from build123d import *

# Parameters (mm, degrees)
PAD014_DEPTH         = 3
SKETCH055_R          = 1.7
POCKET019_DEPTH      = 364.282338
POCKET019_DEPTH_BACK = 367.282338


with BuildPart() as part:
    # Sketch052 → Pad014 (new body)
    with BuildSketch(Plane.XY):
        with BuildLine():
            ThreePointArc((152.959511, 127.101705), (84.480895, 180.040089), (0, 198.875477))
            Line((0, 198.875477), (0, 208.875477))
            ThreePointArc((160.650731, 133.492724), (88.728824, 189.092995), (0, 208.875477))
            ThreePointArc((152.959511, 127.101705), (160.000631, 126.451604), (160.650731, 133.492724))
        make_face()
    pad014 = extrude(amount=PAD014_DEPTH)

    # Sketch055 → Pocket019 (cut, two sides)
    with BuildSketch(Plane.XY) as pocket019_sk:
        with Locations((143.11, 145.205847)):
            Circle(SKETCH055_R)
        with BuildLine():
            Line((0, 202.175477), (0, 205.575477))
            ThreePointArc((0, 202.175477), (1.7, 203.875477), (0, 205.575477))
        make_face()
    pocket019 = extrude(amount=-POCKET019_DEPTH, mode=Mode.SUBTRACT) + extrude(pocket019_sk.sketch, amount=POCKET019_DEPTH_BACK, mode=Mode.SUBTRACT)

    # Mirrored019: Pad014, Pocket019 across Sketch052 V_Axis
    add(pad014.mirror(Plane(origin=(0, 0, 0), x_dir=(0, 0, 1), z_dir=(1, 0, 0))))
    add(pocket019.mirror(Plane(origin=(0, 0, 0), x_dir=(0, 0, 1), z_dir=(1, 0, 0))), mode=Mode.SUBTRACT)


solid = part.part
Geometry: final body of the model. Coordinates: model frame, mm. Round coordinates to 2 decimals unless told otherwise and drop trailing zeros. Loops run counter-clockwise (first coordinate to the right, second up) from the corner with the lowest first, then second, coordinate; pieces in that order, holes last. Notation, with made-up numbers: (17.25, -30.5) -> (26.25, -30.5) arc R26 cw to (26.25, -2.5) -> close; hole circle Ø7 at (86.25, 25). An arc over 180 degrees is marked (long way). One line per question, with ' | ' between items. Start each with the question number.
1. Section D-D on x = -125. Output: boundary loops of the cut face in (y, z), and give its area (3 significant figures).
2. Mould query, pull axis X, two halves, no side actions, for faces 1 (the face through (159.915, 126.382, 1.479)), 2 (the face through (-1, 201, 0)). Classes: pulls with the +X half, pulls with the -X half, needs draft (parallel to the pull), parting line crosses it, or undercut.
3. Section A-A on y = 188.5. Output: boundary loops of the cut face in (x, z), and give its area (3 significant figures).
4. Contact query for flat-ended pins moving along their axis: pin 1 (3 mm diameter, centred on x = 143.11, y = 145.21, fed in from -Z); pin 2 (1.5 mm diameter, centred on x = 110.5, z = 1, fed in from +Y). Output: stop coordinate, or through.
5. Section B-B on z = 0.65. Output: boundary loops of the cut face in (x, y).
6. Line query: line 1 along Y through (x, z) = (0, 0.95); line 2 along Y through (x, z) = (-143.11, 2); line 3 along X through (y, z) = (146, 2.45). Output: solid intervals per line, ascending. Write a range as [from, to].
7. Section C-C on x = -64.5. Output: boundary loops of the cut face in (y, z), and give its area (3 significant figures).
Returned:
1) outline: (154.68, 0) -> (167.34, 0) -> (167.34, 3) -> (154.68, 3) -> close | area: 38.0 mm2
2) face 1: undercut | face 2: needs draft
3) outline: (-89.98, 0) -> (-63.4, 0) -> (-63.4, 3) -> (-89.98, 3) -> close; (63.4, 0) -> (89.98, 0) -> (89.98, 3) -> (63.4, 3) -> close | area: 160 mm2
4) pin 1: passes through | pin 2: stops at y = 177.72
5) outline: (-160.65, 133.49) arc R5 ccw to (-152.96, 127.1) arc R198.88 cw to (0, 198.88) arc R198.88 cw to (152.96, 127.1) arc R5 ccw to (160.65, 133.49) arc R208.88 ccw to (0, 208.88) arc R208.88 ccw to start; hole circle Ø3.4 at (-143.11, 145.21); hole circle Ø3.4 at (0, 203.88); hole circle Ø3.4 at (143.11, 145.21)
6) line 1: y = [198.88, 202.18], [205.58, 208.88] | line 2: y = [138.1, 143.51], [146.91, 152.15] | line 3: x = [-149.38, -144.61], [-141.61, -135.04], [135.04, 141.61], [144.61, 149.38]
7) outline: (188.13, 0) -> (198.67, 0) -> (198.67, 3) -> (188.13, 3) -> close | area: 31.6 mm2
